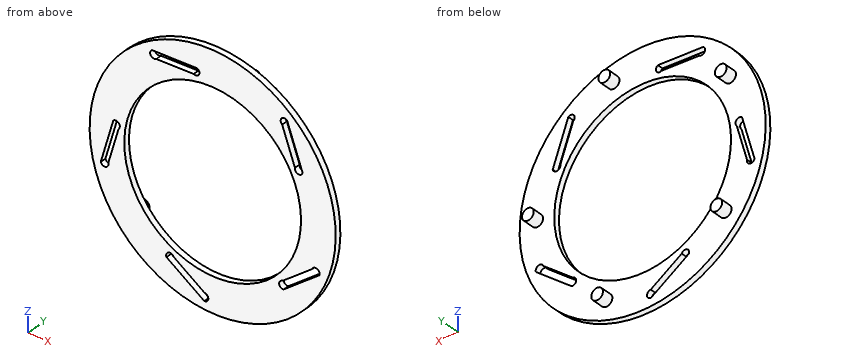
```python
from build123d import *

# Parameters (mm, degrees)
SKETCH1_R           = 31.5
SKETCH1_R_2         = 22.625
BOSS_EXTRUDE1_DEPTH = 1.5
SKETCH2_R           = 1.5
BOSS_EXTRUDE2_DEPTH = 3


with BuildPart() as part:
    # Sketch1 → Boss-Extrude1 (new body)
    with BuildSketch(Plane(origin=(0, 0, 0), x_dir=(1, 0, 0), z_dir=(0, 1, 0))):
        with Locations(Location((0, 0, 0), (0, 0, 270))):
            Circle(SKETCH1_R)
        with Locations(Location((0, 0, 0), (0, 0, 270))):
            Circle(SKETCH1_R_2, mode=Mode.SUBTRACT)
        with BuildLine():
            Line((25.445602695, 10.437123544), (17.907280569, 16.334544855))
            ThreePointArc((17.907280569, 16.334544855), (17.026861096, 17.44127949), (18.13359573, 18.321698963))
            Line((18.13359573, 18.321698963), (27.319881621, 11.135033644))
            ThreePointArc((27.319881621, 11.135033644), (26.731697208, 9.848939131), (25.445602695, 10.437123544))
        make_face(mode=Mode.SUBTRACT)
        with BuildLine():
            Line((-11.821381939, 22.907790728), (-2.147738601, 29.423666069))
            ThreePointArc((-2.147738601, 29.423666069), (-1.106349013, 28.466844389), (-2.063170693, 27.425454801))
            Line((-2.063170693, 27.425454801), (-10.001421306, 22.07848783))
            ThreePointArc((-10.001421306, 22.07848783), (-11.326053072, 21.583158963), (-11.821381939, 22.907790728))
        make_face(mode=Mode.SUBTRACT)
        with BuildLine():
            Line((17.789418023, -20.974957706), (21.068729344, -11.983183919))
            ThreePointArc((21.068729344, -11.983183919), (21.849231951, -10.803855431), (23.028560438, -11.584358037))
            Line((23.028560438, -11.584358037), (19.032354011, -22.541836811))
            ThreePointArc((19.032354011, -22.541836811), (17.627446465, -22.379865253), (17.789418023, -20.974957706))
        make_face(mode=Mode.SUBTRACT)
        with BuildLine():
            Line((-14.451137717, -23.400360319), (-4.886089735, -23.74055981))
            ThreePointArc((-4.886089735, -23.74055981), (-3.523293122, -24.118429356), (-3.901162667, -25.481225968))
            Line((-3.901162667, -25.481225968), (-15.557239956, -25.066654962))
            ThreePointArc((-15.557239956, -25.066654962), (-15.837336158, -23.680456521), (-14.451137717, -23.400360319))
        make_face(mode=Mode.SUBTRACT)
        with BuildLine():
            Line((-26.720712308, 6.51273968), (-24.088498872, -2.689288956))
            ThreePointArc((-24.088498872, -2.689288956), (-24.026746852, -4.102153666), (-25.439611562, -4.163905686))
            Line((-25.439611562, -4.163905686), (-28.647257075, 7.04979206))
            ThreePointArc((-28.647257075, 7.04979206), (-27.415458501, 7.744538254), (-26.720712308, 6.51273968))
        make_face(mode=Mode.SUBTRACT)
    extrude(amount=BOSS_EXTRUDE1_DEPTH)

    # Sketch2 → Boss-Extrude2 (add)
    with BuildSketch(Plane(origin=(0, 1.5, 0), x_dir=(1, 0, 0), z_dir=(0, 1, 0))):
        with Locations(Location((-21.264622422, 16.637783303, 0), (0, 0, 270))):
            Circle(SKETCH2_R)
        with Locations(Location((9.252342519, 25.365215511, 0), (0, 0, 270))):
            Circle(SKETCH2_R)
        with Locations(Location((26.982884575, -0.961217985, 0), (0, 0, 270))):
            Circle(SKETCH2_R)
        with Locations(Location((7.423997262, -25.959280896, 0), (0, 0, 270))):
            Circle(SKETCH2_R)
        with Locations(Location((-22.394601934, -15.082499932, 0), (0, 0, 270))):
            Circle(SKETCH2_R)
    extrude(amount=BOSS_EXTRUDE2_DEPTH)


solid = part.part
```
Check sheet for the modelled part. Datum: model origin and axes. Units: mm. Round coordinates to 2 decimals unless told otherwise and drop trailing zeros. Write each loop counter-clockwise with the first axis right and the second up, starting at its lowest first coordinate (ties: lowest second). Pieces come first, ordered by that corner, then holes. Notation, with made-up numbers: (59, -34) -> (65, -34) arc R29 cw to (65, 2) -> close; hole circle Ø11 at (64.5, 59.25). An arc over 180 degrees is marked (long way). One line per question, with ' | ' between items. Start each with the question number.
1. Scan lines: line 1 along X through (y, z) = (0.8, 0) (3 decimals); line 2 along X through (y, z) = (0.35, -15.5); line 3 along Z through (x, y) = (-2.5, 0.4). Record each from-to range of solid material in increasing order. Write a range as from..to.
2. Sectioned sample at C-C, the plane z = -25. Record the cut outline in (x, y).
3. Sectioned sample at D-D, the plane x = -18. Record the cut outline in (y, z).
4. Depth check by flat-ended pin: pin 1 (2 mm diameter, centred on x = -5.5, y = 1.5, fed in from +Z). Enter the tip coordinate at first touch or a pass-through.
5. Sectioned sample at B-B, the plane y = 3.7. Record the cut outline in (x, z), then the cut area to 3 significant figures.
6. Sectioned sample at A-A, the plane x = 0. Record the cut outline in (y, z) (3 decimals).
Taken from the geometry:
1) line 1: x = -31.5..-26.631, -24.858..-22.625, 22.625..31.5 | line 2: x = -27.42..-16.48, 16.48..18.97, 21.74..27.42 | line 3: z = -31.4..-29.19, -27.13..-22.49, 22.49..31.4
2) outline: (-19.16, 0) -> (-8.72, 0) -> (-8.72, 1.5) -> (-19.16, 1.5) -> close; (-5.66, 0) -> (19.16, 0) -> (19.16, 1.5) -> (10.71, 1.5) -> (10.71, 4.5) -> (7.8, 4.5) -> (7.8, 1.5) -> (-5.66, 1.5) -> close
3) outline: (0, -25.85) -> (1.5, -25.85) -> (1.5, -13.71) -> (0, -13.71) -> close; (0, 13.71) -> (1.5, 13.71) -> (1.5, 25.85) -> (0, 25.85) -> close
4) pin 1: stops at z = 31.18
5) outline: circle Ø3 at (-22.39, 15.08); circle Ø3 at (-21.26, -16.64); circle Ø3 at (7.42, 25.96); circle Ø3 at (9.25, -25.37); circle Ø3 at (26.98, 0.96) | area: 35.3 mm^2
6) outline: (0, -31.5) -> (1.5, -31.5) -> (1.5, -22.625) -> (0, -22.625) -> close; (0, 22.625) -> (1.5, 22.625) -> (1.5, 31.5) -> (0, 31.5) -> close
